```python
from build123d import *

# Parameters (mm, degrees)
F1_DEPTH     = 12.7
F2_T1_DEPTH  = 61.4894192219
F2_T3_DEPTH  = 60.6595144669
F2_T5_DEPTH  = 37.4346345762
F2_T10_DEPTH = 60.8311166964
F2_T15_ANGLE = 160.5521212616
F2_T20_DEPTH = 60.8311166964
F2_T25_ANGLE = 160.5521212616


# Not quite as in the source:
# - a fillet or chamfer that OpenCascade refuses, or shapes differently, is made with other operations: its cross-section is extruded or revolved along the edge and cut away or added


with BuildPart() as f1:
    # F0 (on Top) → F1 (new body)
    with BuildSketch(Plane.XY):
        with BuildLine():
            Line((38.2788181305, 17.8758297116), (42.2920919955, 24.7220024467))
            Line((42.2920919955, 24.7220024467), (42.2820188105, 32.8584946692))
            ThreePointArc((42.2820188105, 32.8584946692), (42.9440997072, 34.690736549), (44.6269139647, 35.6723666191))
            Line((44.6269139647, 35.6723666191), (44.4705858827, 31.9205336273))
            ThreePointArc((44.4705858827, 31.9205336273), (45.6310728705, 34.6386150419), (48.3005791903, 35.9068550169))
            Line((48.3005791903, 35.9068550169), (48.3005791903, 32.4676781893))
            ThreePointArc((48.3005791903, 32.4676781893), (48.8348924642, 30.7225209157), (50.2546578646, 29.5756421983))
            Line((50.2546578646, 29.5756421983), (49.394864589, 28.2468684018))
            ThreePointArc((49.394864589, 28.2468684018), (47.3924953639, 25.9852736124), (44.8100380599, 24.4183633476))
            Line((44.8100380599, 24.4183633476), (44.98494789, 18.4131488204))
            ThreePointArc((44.98494789, 18.4131488204), (47.8016399203, 19.8157230834), (49.7074984014, 22.3194546998))
            Line((49.7074984014, 22.3194546998), (59.6794784069, 44.5563644171))
            Line((59.6794784069, 44.5563644171), (44.9269972742, 75.77765733))
            Line((44.9269972742, 75.77765733), (44.417835772, 72.9466155171))
            ThreePointArc((44.417835772, 72.9466155171), (43.8763497816, 72.371486937), (43.8214614987, 71.5834721923))
            ThreePointArc((43.8214614987, 71.5834721923), (44.9290145189, 72.6595413512), (46.036567539, 71.5834721923))
            Line((46.036567539, 71.5834721923), (49.4444258511, 58.1224299967))
            ThreePointArc((49.4444258511, 58.1224299967), (49.4311906391, 56.2537383436), (48.5072657466, 54.6293780208))
            Line((48.5072657466, 54.6293780208), (47.3145134747, 52.8402514756))
            Line((47.3145134747, 52.8402514756), (48.6776567996, 53.0106425285))
            ThreePointArc((48.6776567996, 53.0106425285), (49.4221984033, 52.9229745419), (50.0408001244, 52.4994656444))
            Line((50.0408001244, 52.4994656444), (52.3411072791, 45.2577620745))
            ThreePointArc((52.3411072791, 45.2577620745), (49.496534757, 43.1348395296), (46.2921559811, 44.6613878012))
            Line((46.2921559811, 44.6613878012), (48.2516773045, 46.5357117355))
            Line((48.2516773045, 46.5357117355), (46.5477481484, 46.7913001776))
            ThreePointArc((46.5477481484, 46.7913001776), (45.0495064909, 45.3175304922), (43.9066551626, 43.5538366437))
            Line((43.9066551626, 43.5538366437), (44.5030331612, 45.6837452948))
            ThreePointArc((44.5030331612, 45.6837452948), (43.1415749719, 44.952040155), (42.2027260065, 43.7242276967))
            ThreePointArc((42.2027260065, 43.7242276967), (41.3363207449, 45.5819979858), (39.9024225771, 47.0468886197))
            ThreePointArc((39.9024225771, 47.0468886197), (37.9368947907, 49.8661923797), (40.2432084084, 52.4142682552))
            ThreePointArc((40.2432084084, 52.4142682552), (43.2781651475, 54.2049845256), (44.6734242141, 57.4408583343))
            ThreePointArc((44.6734242141, 57.4408583343), (43.1144375969, 60.6332712401), (39.817225188, 61.9562715292))
            Line((39.817225188, 61.9562715292), (42.6287092268, 64.767755568))
            Line((42.6287092268, 64.767755568), (38.113296032, 64.0861839056))
            Line((38.113296032, 64.0861839056), (36.9205437601, 69.0275803208))
            Line((36.9205437601, 69.0275803208), (36.1537747085, 64.5121708512))
            Line((36.1537747085, 64.5121708512), (35.046223551, 62.0414689183))
            Line((35.046223551, 62.0414689183), (35.3018119931, 60.2523423731))
            Line((35.3018119931, 60.2523423731), (34.1090597212, 58.8891990483))
            Line((34.1090597212, 58.8891990483), (35.216614604, 57.0148788393))
            ThreePointArc((35.216614604, 57.0148788393), (36.4787140011, 59.9990779117), (39.6468304098, 60.6783255935))
            ThreePointArc((39.6468304098, 60.6783255935), (42.100861171, 59.7637799228), (43.3102808893, 57.4408583343))
            ThreePointArc((43.3102808893, 57.4408583343), (41.960859951, 55.6347382447), (39.987616241, 54.5441806316))
            Line((39.987616241, 54.5441806316), (37.5169217587, 53.521823138))
            ThreePointArc((37.5169217587, 53.521823138), (35.2577529504, 50.8211890197), (35.1314172149, 47.302480787))
            Line((35.1314172149, 47.302480787), (36.494564265, 43.8946224749))
            ThreePointArc((36.494564265, 43.8946224749), (35.5191674638, 45.2611219807), (34.0238660574, 46.024531126))
            Line((34.0238660574, 46.024531126), (33.9386686683, 44.4057993591))
            ThreePointArc((33.9386686683, 44.4057993591), (32.5250680188, 45.9137846149), (30.6160058826, 46.7061027884))
            ThreePointArc((30.6160058826, 46.7061027884), (31.4840333326, 45.4817930881), (31.9791510701, 44.0650135279))
            ThreePointArc((31.9791510701, 44.0650135279), (29.0027298162, 43.1420138964), (26.4413785189, 44.9169762433))
            Line((26.4413785189, 44.9169762433), (28.2305050641, 52.5846593082))
            ThreePointArc((28.2305050641, 52.5846593082), (30.0752112346, 52.9015778311), (31.3827730715, 51.5623018146))
            Line((31.3827730715, 51.5623018146), (31.6383615136, 53.0958399177))
            ThreePointArc((31.6383615136, 53.0958399177), (30.9888271445, 53.8193992901), (30.1900226623, 54.3737858534))
            ThreePointArc((30.1900226623, 54.3737858534), (29.5328449453, 55.9706841256), (29.593648389, 57.6964505017))
            Line((29.593648389, 57.6964505017), (32.9163111746, 70.8167105913))
            ThreePointArc((32.9163111746, 70.8167105913), (33.7093855935, 71.7795807909), (34.7906313837, 71.1574926972))
            ThreePointArc((34.7906313837, 71.1574926972), (34.7651749092, 72.4631986698), (33.5519872606, 72.9466155171))
            Line((33.5519872606, 72.9466155171), (33.5519872606, 76.6831859946))
            Line((33.5519872606, 76.6831859946), (18.7778156251, 44.5563644171))
            Line((18.7778156251, 44.5563644171), (33.3570353687, 13.0645893514))
            Line((33.3570353687, 13.0645893514), (33.3570353687, 24.4183633476))
            ThreePointArc((33.3570353687, 24.4183633476), (30.754145435, 26.167413579), (29.0718954057, 28.8139674813))
            ThreePointArc((29.0718954057, 28.8139674813), (29.8771193905, 32.3095735456), (29.9375038594, 35.8962155879))
            ThreePointArc((29.9375038594, 35.8962155879), (32.545088234, 34.1789060872), (33.6360111833, 31.2534086406))
            ThreePointArc((33.6360111833, 31.2534086406), (34.5240159071, 33.128980926), (34.2655442655, 35.1879894733))
            ThreePointArc((34.2655442655, 35.1879894733), (38.2849845666, 30.6609560826), (39.4591912627, 24.7220024467))
            Line((39.4591912627, 24.7220024467), (35.996761173, 17.8758297116))
            Line((35.996761173, 17.8758297116), (37.8066673875, 13.705172576))
            Line((37.8066673875, 13.705172576), (34.8163843155, 9.3771321699))
            Line((34.8163843155, 9.3771321699), (39.2231196165, 0))
            Line((39.2231196165, 0), (42.4494743347, 7.9606827348))
            ThreePointArc((42.4494743347, 7.9606827348), (38.9638620653, 6.181357436), (36.7049872875, 9.3771321699))
            Line((36.7049872875, 9.3771321699), (39.2231196165, 13.705172576))
            Line((39.2231196165, 13.705172576), (38.2788181305, 17.8758297116))
        make_face()
    extrude(amount=F1_DEPTH)

    # F2: chamfer of 5.08 on 10 edges, made by hand

    # F2_s2 → F2_t1 (cut)
    with BuildSketch(Plane(origin=(40.423720467, 87.9024345312, 0), x_dir=(0, 0, 1), z_dir=(-0.4178083615, -0.9085351799, 0))):
        Polygon((7.62, 1.5557155161), (12.7, -3.5242844839), (12.7, 1.5557155161), align=None)
        Polygon((5.08, 1.5557155161), (0, -3.5242844839), (0, 1.5557155161), align=None)
    extrude(amount=F2_T1_DEPTH, mode=Mode.SUBTRACT)

    # F2_s4 → F2_t3 (cut)
    with BuildSketch(Plane(origin=(-0.736952526, 1.5596434572, 0), x_dir=(0, 0, 1), z_dir=(-0.4272216023, 0.9041469474, 0))):
        Polygon((7.62, 72.9944596236), (12.7, 67.9144596236), (12.7, 72.9944596236), align=None)
        Polygon((5.08, 72.9944596236), (0, 67.9144596236), (0, 72.9944596236), align=None)
    extrude(amount=F2_T3_DEPTH, mode=Mode.SUBTRACT)

    # F2_s6 → F2_t5 (cut)
    with BuildSketch(Plane(origin=(16.6557348467, 37.141277044, 0), x_dir=(0, 0, 1), z_dir=(0.4091826653, 0.91245249, 0))):
        Polygon((7.62, 36.2229967242), (12.7, 31.1429967242), (12.7, 36.2229967242), align=None)
        Polygon((5.08, 36.2229967242), (0, 31.1429967242), (0, 36.2229967242), align=None)
    extrude(amount=F2_T5_DEPTH, mode=Mode.SUBTRACT)


with BuildPart() as f2_tool8:
    # F2_s9 → F2_t10 (new body)
    with BuildSketch(Plane(origin=(-19.1610255807, 41.3886832236, 0), x_dir=(0, 0, 1), z_dir=(0.4201163127, -0.9074702661, 0))):
        Polygon((7.62, -35.7591648667), (12.7, -40.8391648667), (12.7, -35.7591648667), align=None)
    extrude(amount=F2_T10_DEPTH)

    split(bisect_by=Plane(origin=(21.465639244, -10.8561787862, 0), x_dir=(0, 0, 1), z_dir=(-0.8923664741, 0.4513115065, 0)), keep=Keep.TOP)


with BuildPart() as f1_1:
    add(f1.part)

    # F2_t7: cut F2_tool8
    add(f2_tool8.part, mode=Mode.SUBTRACT)


with BuildPart() as f2_tool13:
    # F2_s14 → F2_t15 (revolve)
    with BuildSketch(Plane(origin=(2.3486048787, 28.532346778, 0), x_dir=(0, 0, 1), z_dir=(0.0820363131, 0.996629341, 0))):
        Polygon((7.62, 34.2474692794), (12.7, 39.3274692794), (12.7, 34.2474692794), align=None)
    revolve(axis=Axis((43.3856729768, 25.154431211, 12.7), (0, 0, 1)), revolution_arc=F2_T15_ANGLE)

    split(bisect_by=Plane(origin=(45.4826703508, 1.3247430391, 0), x_dir=(0, 0, 1), z_dir=(0.9995760983, 0.0291139783, 0)), keep=Keep.TOP)


with BuildPart() as f1_2:
    add(f1_1.part)

    # F2_t12: cut F2_tool13
    add(f2_tool13.part, mode=Mode.SUBTRACT)


with BuildPart() as f2_tool18:
    # F2_s19 → F2_t20 (new body)
    with BuildSketch(Plane(origin=(-19.1610255807, 41.3886832236, 0), x_dir=(0, 0, 1), z_dir=(0.4201163127, -0.9074702661, 0))):
        Polygon((5.08, -35.7591648667), (0, -40.8391648667), (0, -35.7591648667), align=None)
    extrude(amount=F2_T20_DEPTH)

    split(bisect_by=Plane(origin=(21.465639244, -10.8561787862, 0), x_dir=(0, 0, 1), z_dir=(-0.8923664741, 0.4513115065, 0)), keep=Keep.TOP)


with BuildPart() as f1_3:
    add(f1_2.part)

    # F2_t17: cut F2_tool18
    add(f2_tool18.part, mode=Mode.SUBTRACT)


with BuildPart() as f2_tool23:
    # F2_s24 → F2_t25 (revolve)
    with BuildSketch(Plane(origin=(2.3486048787, 28.532346778, 0), x_dir=(0, 0, 1), z_dir=(0.0820363131, 0.996629341, 0))):
        Polygon((5.08, 34.2474692794), (0, 39.3274692794), (0, 34.2474692794), align=None)
    revolve(axis=Axis((43.3856729768, 25.154431211, 0), (0, 0, 1)), revolution_arc=F2_T25_ANGLE)

    split(bisect_by=Plane(origin=(45.4826703508, 1.3247430391, 0), x_dir=(0, 0, 1), z_dir=(0.9995760983, 0.0291139783, 0)), keep=Keep.TOP)


with BuildPart() as f1_4:
    add(f1_3.part)

    # F2_t22: cut F2_tool23
    add(f2_tool23.part, mode=Mode.SUBTRACT)


solid = f1_4.part
```
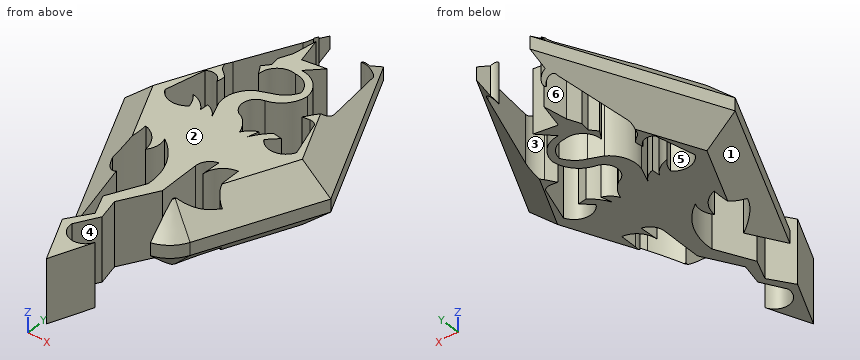
Geometry: final body of the model. Coordinates: model frame, mm. Face numbers are marked on the shaded views. A direction names the side the tool comes from. Coordinates: 2 decimals unless noted, no trailing zeros. Order: outer loops, then holes, each group sorted by start corner. A loop starts at its lowest first (then second) coordinate and runs counter-clockwise, first axis right, second up. Notation, with made-up numbers: (71, 7.25) -> (102, 7.25) arc R19 ccw to (102, 39.25) -> close; hole circle Ø2 at (-36.75, 88.25). An arc over 180 degrees is marked (long way). Use CSV: the item, a comma, the result in double quotes.
1) Line query: line 1 (Y direction, x = 41, z = 7.75); line 2 (X direction, y = 35, z = 4.25); line 3 (X direction, y = 28.5, z = 6.5). Output: solid intervals per line, ascending.
Findings:
line 1,"y = 4.38 to 6.4, 22.52 to 46.02, 52.64 to 54.97, 60.43 to 61.8, 63.14 to 64.52"
line 2,"x = 24.12 to 29.99, 31.72 to 34.34, 34.54 to 43.24, 44.6 to 46.03, 48.3 to 54.48"
line 3,"x = 26.21 to 29.2, 39.1 to 42.29, 49.56 to 52.48"
2) Pin query (flat end, axial travel): pin 1 Ø4 at (x, y) = (51, 18) entering from +Z; pin 2 Ø1.1 at (y, z) = (74.5, 6) entering from +X; pin 3 Ø12 at (x, y) = (39.5, 35) entering from -Z; pin 4 Ø4 at (y, z) = (58, 10.5) entering from +X. Return the tip coordinate at first contact, or that it passes through.
Findings:
pin 1,"passes through"
pin 2,"stops at x = 45.79"
pin 3,"stops at z = 0"
pin 4,"stops at x = 52.55"
3) Section A-A on y = 37.5. Output: boundary loops of the cut face in (x, z).
Findings:
outline,"(22.04, 5.08) -> (27.64, 0) -> (50.95, 0) -> (56.52, 5.08) -> (56.52, 7.62) -> (50.95, 12.7) -> (27.64, 12.7) -> (22.04, 7.62) -> close"
4) Mould query, pull axis X, two halves, no side actions, for the marked faces 1, 2 and 3. Classes: +X half, -X half, draft (parallel to the pull), parting line (faces both ways), or undercut.
Findings:
face 1,"-X half"
face 2,"draft"
face 3,"undercut"
5) Access query for the marked faces 4, 5 and 6. Directions: +Z, -Z, +X, -X, +Y, -Y. A direction counts if a zero-diameter tool reaches every point of the face in a straight line with its end or side. Return the directions, or none.
Findings:
face 4,"+Z, -Z, +X"
face 5,"+Z, -Z"
face 6,"+Z, -Z, +Y"
